from build123d import *

# Parameters (mm, degrees)
SKETCH1_W           = 50
SKETCH1_H           = 50
BOSS_EXTRUDE1_DEPTH = 3
SKETCH2_W           = 50
SKETCH2_H           = 3
BOSS_EXTRUDE2_DEPTH = 47
BOSS_EXTRUDE3_DEPTH = 1.5
CUT_EXTRUDE1_REACH  = 52
SKETCH4_R           = 1.9
SKETCH4_W           = 7.5
SKETCH4_H           = 7.5
FILLET1_R           = 1
CUT_EXTRUDE3_DEPTH  = 1
BOSS_EXTRUDE4_DEPTH = 2
FILLET3_R           = 3
CUT_EXTRUDE4_REACH  = 5
SKETCH8_R           = 2.25


with BuildPart() as part:
    # Sketch1 → Boss-Extrude1 (new body)
    with BuildSketch(Plane(origin=(0, 0, 0), x_dir=(1, 0, 0), z_dir=(0, 1, 0))):
        Rectangle(SKETCH1_W, SKETCH1_H)
    extrude(amount=BOSS_EXTRUDE1_DEPTH)

    # Sketch2 → Boss-Extrude2 (add)
    with BuildSketch(Plane(origin=(0, 3, 0), x_dir=(1, 0, 0), z_dir=(0, 1, 0))):
        with Locations((0, 23.5)):
            Rectangle(SKETCH2_W, SKETCH2_H)
    extrude(amount=BOSS_EXTRUDE2_DEPTH)

    # Sketch3 → Boss-Extrude3 (add, symmetric)
    with BuildSketch(Plane(origin=(0, 0, 0), x_dir=(0, 0, -1), z_dir=(1, 0, 0))):
        Polygon((-25, 3), (22, 50), (22, 3), align=None)
    extrude(amount=BOSS_EXTRUDE3_DEPTH, both=True)

    # Sketch4 → Cut-Extrude1 (cut, up to next)
    with BuildSketch(Plane(origin=(0, 0, -25), x_dir=(-1, 0, 0), z_dir=(0, 0, -1)), mode=Mode.PRIVATE) as cut_extrude1_sk1:
        with Locations((-18.425, 17.5)):
            Circle(SKETCH4_R)
    cut_extrude1_tool1 = extrude(cut_extrude1_sk1.sketch, amount=-CUT_EXTRUDE1_REACH, mode=Mode.PRIVATE) & part.part
    add(cut_extrude1_tool1.solids().sort_by_distance((18.425, 17.5, -25))[0], mode=Mode.SUBTRACT)
    # Sketch4 → Cut-Extrude1 (cut, up to next)
    with BuildSketch(Plane(origin=(0, 0, -25), x_dir=(-1, 0, 0), z_dir=(0, 0, -1)), mode=Mode.PRIVATE) as cut_extrude1_sk2:
        with Locations((18.425, 17.5)):
            Circle(SKETCH4_R)
    cut_extrude1_tool2 = extrude(cut_extrude1_sk2.sketch, amount=-CUT_EXTRUDE1_REACH, mode=Mode.PRIVATE) & part.part
    add(cut_extrude1_tool2.solids().sort_by_distance((-18.425, 17.5, -25))[0], mode=Mode.SUBTRACT)
    # Sketch4 → Cut-Extrude1 (cut, up to next)
    with BuildSketch(Plane(origin=(0, 0, -25), x_dir=(-1, 0, 0), z_dir=(0, 0, -1)), mode=Mode.PRIVATE) as cut_extrude1_sk3:
        with Locations((9.5, 15)):
            Rectangle(SKETCH4_W, SKETCH4_H)
    cut_extrude1_tool3 = extrude(cut_extrude1_sk3.sketch, amount=-CUT_EXTRUDE1_REACH, mode=Mode.PRIVATE) & part.part
    add(cut_extrude1_tool3.solids().sort_by_distance((-9.5, 15, -25))[0], mode=Mode.SUBTRACT)

    # Fillet1
    fillet1_edges = [part.edges().sort_by_distance(p)[0] for p in [
        (-13.25, 18.75, -23.5),
        (-13.25, 11.25, -23.5),
        (-5.75, 11.25, -23.5),
        (-5.75, 18.75, -23.5),
    ]]
    fillet(fillet1_edges, radius=FILLET1_R)

    # Sketch6 → Cut-Extrude3 (cut)
    with BuildSketch(Plane.XY.offset(-22)):
        Polygon((16.779551733, 14.65), (20.070448267, 14.65), (21.715896534, 17.5), (20.070448267, 20.35), (16.779551733, 20.35), (15.134103466, 17.5), align=None)
        Polygon((-20.070448267, 14.65), (-21.715896534, 17.5), (-20.070448267, 20.35), (-16.779551733, 20.35), (-15.134103466, 17.5), (-16.779551733, 14.65), align=None)
    extrude(amount=-CUT_EXTRUDE3_DEPTH, mode=Mode.SUBTRACT)

    # Sketch7 → Boss-Extrude4 (add)
    with BuildSketch(Plane.XY.offset(-22)):
        Polygon((-15.913526329, 13.15), (-13.402052658, 17.5), (-15.913526329, 21.85), (-20.936473671, 21.85), (-23.447947342, 17.5), (-20.936473671, 13.15), align=None)
        Polygon((-16.779551733, 14.65), (-15.134103466, 17.5), (-16.779551733, 20.35), (-20.070448267, 20.35), (-21.715896534, 17.5), (-20.070448267, 14.65), align=None, mode=Mode.SUBTRACT)
        Polygon((13.402052658, 17.5), (15.913526329, 13.15), (20.936473671, 13.15), (23.447947342, 17.5), (20.936473671, 21.85), (15.913526329, 21.85), align=None)
        Polygon((16.779551733, 14.65), (20.070448267, 14.65), (21.715896534, 17.5), (20.070448267, 20.35), (16.779551733, 20.35), (15.134103466, 17.5), align=None, mode=Mode.SUBTRACT)
    extrude(amount=BOSS_EXTRUDE4_DEPTH)

    # Fillet3
    fillet3_edges = [part.edges().sort_by_distance(p)[0] for p in [
        (-13.25, 3, -22),
        (-25, 50, -23.5),
        (25, 50, -23.5),
        (13.25, 3, -22),
        (25, 1.5, 25),
        (-25, 1.5, 25),
    ]]
    fillet(fillet3_edges, radius=FILLET3_R)

    # Sketch8 → Cut-Extrude4 (cut, up to next)
    with BuildSketch(Plane(origin=(0, 3, 0), x_dir=(1, 0, 0), z_dir=(0, 1, 0)), mode=Mode.PRIVATE) as cut_extrude4_sk1:
        with Locations((-13.25, 0)):
            Circle(SKETCH8_R)
    cut_extrude4_tool1 = extrude(cut_extrude4_sk1.sketch, amount=-CUT_EXTRUDE4_REACH, mode=Mode.PRIVATE) & part.part
    add(cut_extrude4_tool1.solids().sort_by_distance((-13.25, 3, 0))[0], mode=Mode.SUBTRACT)
    # Sketch8 → Cut-Extrude4 (cut, up to next)
    with BuildSketch(Plane(origin=(0, 3, 0), x_dir=(1, 0, 0), z_dir=(0, 1, 0)), mode=Mode.PRIVATE) as cut_extrude4_sk2:
        with Locations((13.25, 0)):
            Circle(SKETCH8_R)
    cut_extrude4_tool2 = extrude(cut_extrude4_sk2.sketch, amount=-CUT_EXTRUDE4_REACH, mode=Mode.PRIVATE) & part.part
    add(cut_extrude4_tool2.solids().sort_by_distance((13.25, 3, 0))[0], mode=Mode.SUBTRACT)


solid = part.part
Verification items for the finished model (mm, model axes). A direction names the side the tool comes from. Give positions to 0.01 mm unless a question says otherwise; leave off trailing zeros. Loops run counter-clockwise (first coordinate to the right, second up) from the corner with the lowest first, then second, coordinate; pieces in that order, holes last.
1. Tool access check on faces 4 (the flat face through (22.21, 19.645, -21.014)), 5 (the flat face through (-18, 14.65, -22)), 6 (the flat face through (-22.17, 19.71, -21.01)). Record the directions out of +Z, -Z, +X, -X, +Y, -Y that give a thin tool (end or side, any length) a straight path to the whole face; none if there is none.
Derived:
face 4: +Z, +X, +Y
face 5: +Z
face 6: +Z, -X, +Y
2. Material ranges on probe 1 along X at (y, z) = (1, 0); probe 2 along Y at (x, z) = (-6, -4); probe 3 along X at (y, z) = (42, -20.5), recorded low to high.
Derived:
probe 1: x = -25 to -15.5, -11 to 11, 15.5 to 25
probe 2: y = 0 to 3
probe 3: x = -1.5 to 1.5
3. Release check for a two-part mould opening along Z. For faces 1 (the flat face through (-16, 16, -22)), 2 (the cylindrical face through (11, 2, 0)), 3 (the cylindrical face through (-13.09, 3.86, -21.1)) record: +Z half, -Z half, draft (parallel to the pull), parting line (faces both ways), or undercut.
Derived:
face 1: draft
face 2: undercut
face 3: +Z half
4. Cross-section at B-B on x = -10. Record the cut outline in (y, z).
Derived:
outline: (0, -25) - (11.25, -25) - (11.25, -22) - (6, -22) arc R3 cw to (3, -19) - (3, 25) - (0, 25) - close; (18.75, -25) - (50, -25) - (50, -22) - (18.75, -22) - close
5. Go/stop test with flat-tipped pins: P1, Ø0.6, axis at x = 19.5, z = -20.5, coming from the +Y side; P2, Ø12, axis at x = 11, z = 7.5, coming from the +Y side; P3, Ø2, axis at y = 23.5, z = -18, coming from the -X side. Record where each tip stops, or that it passes through.
Derived:
P1: stops at y = 21.85
P2: stops at y = 3
P3: stops at x = -1.5
6. Cross-section at A-A on z = 0. Record the cut outline in (x, y), and give its area (3 significant figures).
Derived:
outline: (-25, 0) - (-15.5, 0) - (-15.5, 3) - (-25, 3) - close; (-11, 0) - (11, 0) - (11, 3) - (1.5, 3) - (1.5, 28) - (-1.5, 28) - (-1.5, 3) - (-11, 3) - close; (15.5, 0) - (25, 0) - (25, 3) - (15.5, 3) - close
area: 198 mm2
7. Cross-section at D-D on z = 16.5. Record the cut outline in (x, y).
Derived:
outline: (-25, 0) - (25, 0) - (25, 3) - (1.5, 3) - (1.5, 11.5) - (-1.5, 11.5) - (-1.5, 3) - (-25, 3) - close
8. Cross-section at C-C on y = 39.5. Record the cut outline in (x, z), and give its area (4 significant figures).
Derived:
outline: (-25, -25) - (25, -25) - (25, -22) - (1.5, -22) - (1.5, -11.5) - (-1.5, -11.5) - (-1.5, -22) - (-25, -22) - close
area: 181.5 mm2
